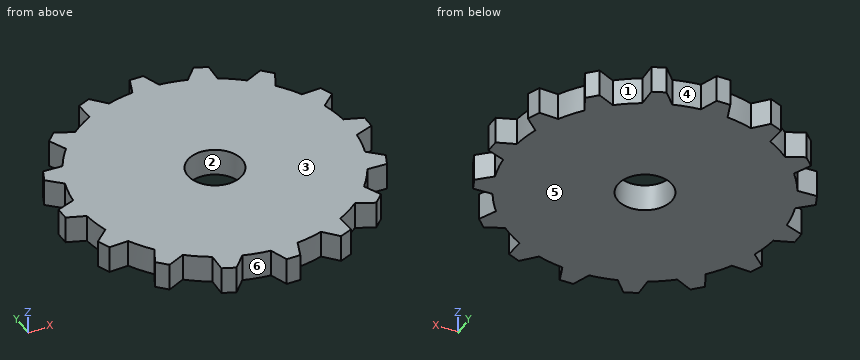
```python
from build123d import *

# Parameters (mm, degrees)
SKETCH2_R           = 1
BOSS_EXTRUDE2_DEPTH = 1


with BuildPart() as part:
    # Sketch2 → Boss-Extrude2 (new body)
    with BuildSketch(Plane.XY):
        with BuildLine():
            Line((-0.25, 5.638363295), (0.25, 5.638363295))
            Line((0.25, 5.638363295), (0.491146384, 4.975819051))
            ThreePointArc((0.491146384, 4.975819051), (0.97545161, 4.903926402), (1.450403422, 4.785010963))
            Line((1.450403422, 4.785010963), (1.926738336, 5.304839303))
            Line((1.926738336, 5.304839303), (2.388678102, 5.113497587))
            Line((2.388678102, 5.113497587), (2.357923605, 4.409103795))
            ThreePointArc((2.357923605, 4.409103795), (2.777851165, 4.157348062), (3.171142455, 3.865728332))
            Line((3.171142455, 3.865728332), (3.810148226, 4.163701616))
            Line((3.810148226, 4.163701616), (4.163701616, 3.810148226))
            Line((4.163701616, 3.810148226), (3.865728332, 3.171142455))
            ThreePointArc((3.865728332, 3.171142455), (4.157348062, 2.777851165), (4.409103795, 2.357923605))
            Line((4.409103795, 2.357923605), (5.113497587, 2.388678102))
            Line((5.113497587, 2.388678102), (5.304839303, 1.926738336))
            Line((5.304839303, 1.926738336), (4.785010963, 1.450403422))
            ThreePointArc((4.785010963, 1.450403422), (4.903926402, 0.97545161), (4.975819051, 0.491146384))
            Line((4.975819051, 0.491146384), (5.638363295, 0.25))
            Line((5.638363295, 0.25), (5.638363295, -0.25))
            Line((5.638363295, -0.25), (4.975819051, -0.491146384))
            ThreePointArc((4.975819051, -0.491146384), (4.903926402, -0.97545161), (4.785010963, -1.450403422))
            Line((4.785010963, -1.450403422), (5.304839303, -1.926738336))
            Line((5.304839303, -1.926738336), (5.113497587, -2.388678102))
            Line((5.113497587, -2.388678102), (4.409103795, -2.357923605))
            ThreePointArc((4.409103795, -2.357923605), (4.157348062, -2.777851165), (3.865728332, -3.171142455))
            Line((3.865728332, -3.171142455), (4.163701616, -3.810148226))
            Line((4.163701616, -3.810148226), (3.810148226, -4.163701616))
            Line((3.810148226, -4.163701616), (3.171142455, -3.865728332))
            ThreePointArc((3.171142455, -3.865728332), (2.777851165, -4.157348062), (2.357923605, -4.409103795))
            Line((2.357923605, -4.409103795), (2.388678102, -5.113497587))
            Line((2.388678102, -5.113497587), (1.926738336, -5.304839303))
            Line((1.926738336, -5.304839303), (1.450403422, -4.785010963))
            ThreePointArc((1.450403422, -4.785010963), (0.97545161, -4.903926402), (0.491146384, -4.975819051))
            Line((0.491146384, -4.975819051), (0.25, -5.638363295))
            Line((0.25, -5.638363295), (-0.25, -5.638363295))
            Line((-0.25, -5.638363295), (-0.491146384, -4.975819051))
            ThreePointArc((-0.491146384, -4.975819051), (-0.97545161, -4.903926402), (-1.450403422, -4.785010963))
            Line((-1.450403422, -4.785010963), (-1.926738336, -5.304839303))
            Line((-1.926738336, -5.304839303), (-2.388678102, -5.113497587))
            Line((-2.388678102, -5.113497587), (-2.357923605, -4.409103795))
            ThreePointArc((-2.357923605, -4.409103795), (-2.777851165, -4.157348062), (-3.171142455, -3.865728332))
            Line((-3.171142455, -3.865728332), (-3.810148226, -4.163701616))
            Line((-3.810148226, -4.163701616), (-4.163701616, -3.810148226))
            Line((-4.163701616, -3.810148226), (-3.865728332, -3.171142455))
            ThreePointArc((-3.865728332, -3.171142455), (-4.157348062, -2.777851165), (-4.409103795, -2.357923605))
            Line((-4.409103795, -2.357923605), (-5.113497587, -2.388678102))
            Line((-5.113497587, -2.388678102), (-5.304839303, -1.926738336))
            Line((-5.304839303, -1.926738336), (-4.785010963, -1.450403422))
            ThreePointArc((-4.785010963, -1.450403422), (-4.903926402, -0.97545161), (-4.975819051, -0.491146384))
            Line((-4.975819051, -0.491146384), (-5.638363295, -0.25))
            Line((-5.638363295, -0.25), (-5.638363295, 0.25))
            Line((-5.638363295, 0.25), (-4.975819051, 0.491146384))
            ThreePointArc((-4.975819051, 0.491146384), (-4.903926402, 0.97545161), (-4.785010963, 1.450403422))
            Line((-4.785010963, 1.450403422), (-5.304839303, 1.926738336))
            Line((-5.304839303, 1.926738336), (-5.113497587, 2.388678102))
            Line((-5.113497587, 2.388678102), (-4.409103795, 2.357923605))
            ThreePointArc((-4.409103795, 2.357923605), (-4.157348062, 2.777851165), (-3.865728332, 3.171142455))
            Line((-3.865728332, 3.171142455), (-4.163701616, 3.810148226))
            Line((-4.163701616, 3.810148226), (-3.810148226, 4.163701616))
            Line((-3.810148226, 4.163701616), (-3.171142455, 3.865728332))
            ThreePointArc((-3.171142455, 3.865728332), (-2.777851165, 4.157348062), (-2.357923605, 4.409103795))
            Line((-2.357923605, 4.409103795), (-2.388678102, 5.113497587))
            Line((-2.388678102, 5.113497587), (-1.926738336, 5.304839303))
            Line((-1.926738336, 5.304839303), (-1.450403422, 4.785010963))
            ThreePointArc((-1.450403422, 4.785010963), (-0.97545161, 4.903926402), (-0.491146384, 4.975819051))
            Line((-0.491146384, 4.975819051), (-0.25, 5.638363295))
        make_face()
        Circle(SKETCH2_R, mode=Mode.SUBTRACT)
    extrude(amount=BOSS_EXTRUDE2_DEPTH)


solid = part.part
```
For this review, take the finished solid that the model builds, in its own axes (mm). Face numbers are marked on the shaded views. A direction names the side the tool comes from. Coordinates: 2 decimals unless noted, no trailing zeros. Order: outer loops, then holes, each group sorted by start corner. A loop starts at its lowest first (then second) coordinate and runs counter-clockwise, first axis right, second up. Notation, with made-up numbers: (-36.75, 13.25) -> (-2.75, 13.25) arc R19 cw to (-2.75, 30.25) -> close; hole circle Ø8 at (-18, 41.25). An arc over 180 degrees is marked (long way). Use CSV: the item, a comma, the result in double quotes. Start each with the question number.
Item 1: Draft analysis for pull direction X (two halves, no side actions). For the marked faces 1, 2 and 3, state which applies: pulls with the +X half, pulls with the -X half, needs draft (parallel to the pull), parting line crosses it, or undercut.
Item 2: We need section C-C, the plane y = -4. Give the boundary of the cut face in (x, z), then the cut area to 3 significant figures.
Item 3: We need section A-A, the plane y = 0. Give the boundary of the cut face in (x, z), then the cut area to 3 significant figures.
Item 4: We need section D-D, the plane x = 1.25. Give the boundary of the cut face in (y, z).
Item 5: Wall thickness on probe 1 along Y at (x, z) = (0, 0.6); probe 2 along X at (y, z) = (1.5, 0.95); probe 3 along X at (y, z) = (-2, 0.25): over which ranges is each line inside the solid? List them lowest first.
Item 6: For the marked faces 4, 5 and 6, list the 3-axis set-ups (+Z, -Z, +X, -X, +Y, -Y) from which the entire face can be reached by the end or side of a thin tool; tool diameter is ignored.
Derived:
1,face 1,"undercut"
1,face 2,"undercut"
1,face 3,"needs draft"
2,outline,"(-3.97, 0) -> (-3.46, 0) -> (-3.46, 1) -> (-3.97, 1) -> close; (-3, 0) -> (3, 0) -> (3, 1) -> (-3, 1) -> close; (3.46, 0) -> (3.97, 0) -> (3.97, 1) -> (3.46, 1) -> close"
2,area,"7.03 mm^2"
3,outline,"(-5.64, 0) -> (-1, 0) -> (-1, 1) -> (-5.64, 1) -> close; (1, 0) -> (5.64, 0) -> (5.64, 1) -> (1, 1) -> close"
3,area,"9.28 mm^2"
4,outline,"(-4.84, 0) -> (4.84, 0) -> (4.84, 1) -> (-4.84, 1) -> close"
5,probe 1,"y = -5.64 to -1, 1 to 5.64"
5,probe 2,"x = -4.84 to 4.84"
5,probe 3,"x = -5.27 to 5.27"
6,face 4,"+Z, -Z, +Y"
6,face 5,"-Z, +X, -X, +Y, -Y"
6,face 6,"+Z, -Z, -Y"
